Autodesk Inventor part; units mm, degrees
ref_plane "Work Plane3" through (0, 0, 250) normal (0, 0, 1) x (1, 0, 0)
ref_plane "Start Plane" through (0, 0, 0) normal (0, 0, 1) x (1, 0, 0)
ref_plane "End Plane" through (0, 0, 450) normal (0, 0, 1) x (1, 0, 0)
sketch "Sketch" plane through (0, 0, 0) normal (0, 0, 1) x (1, 0, 0)
  line L0 (-13, 15) -> (13, 15)
  line L1 (15, 13) -> (15, -13)
  line L2 (-15, 15) -> (15, -15) construction
  line L3 (15, 15) -> (-15, -15) construction
  line L4 (-5.2, 15) -> (-5.2, 14.2)
  line L5 (-5.2, 14.2) -> (-4.1, 14.2)
  line L6 (-4.1, 14.2) -> (-4.1, 12.2)
  line L7 (-4.1, 12.2) -> (-8.25, 12.2)
  line L8 (-8.25, 12.2) -> (-8.25, 10.2)
  line L9 (-8.25, 10.2) -> (-3.85, 5.8)
  line L10 (-3.85, 5.8) -> (3.85, 5.8)
  line L11 (8.25, 12.2) -> (4.1, 12.2)
  line L12 (4.1, 12.2) -> (4.1, 14.2)
  line L13 (4.1, 14.2) -> (5.2, 14.2)
  line L14 (5.2, 14.2) -> (5.2, 15)
  line L15 (8.25, 12.2) -> (8.25, 10.2)
  line L16 (8.25, 10.2) -> (3.85, 5.8)
  line L17 (-2.5, 0) -> (0, 0)
  line L18 (-5.2, -15) -> (-5.2, -14.2)
  line L19 (-5.2, -14.2) -> (-4.1, -14.2)
  line L20 (-4.1, -14.2) -> (-4.1, -12.2)
  line L21 (-4.1, -12.2) -> (-8.25, -12.2)
  line L22 (-8.25, -12.2) -> (-8.25, -10.2)
  line L23 (-8.25, -10.2) -> (-3.85, -5.8)
  line L24 (-3.85, -5.8) -> (3.85, -5.8)
  line L25 (8.25, -12.2) -> (4.1, -12.2)
  line L26 (4.1, -12.2) -> (4.1, -14.2)
  line L27 (4.1, -14.2) -> (5.2, -14.2)
  line L28 (5.2, -14.2) -> (5.2, -15)
  line L29 (8.25, -12.2) -> (8.25, -10.2)
  line L30 (8.25, -10.2) -> (3.85, -5.8)
  line L31 (15, 5.2) -> (14.2, 5.2)
  line L32 (14.2, 5.2) -> (14.2, 4.1)
  line L33 (14.2, 4.1) -> (12.2, 4.1)
  line L34 (12.2, 4.1) -> (12.2, 8.25)
  line L35 (15, -5.2) -> (14.2, -5.2)
  line L36 (14.2, -5.2) -> (14.2, -4.1)
  line L37 (14.2, -4.1) -> (12.2, -4.1)
  line L38 (12.2, -4.1) -> (12.2, -8.25)
  line L39 (12.2, -8.25) -> (10.2, -8.25)
  line L40 (10.2, -8.25) -> (5.8, -3.85)
  line L41 (5.8, -3.85) -> (5.8, 3.85)
  line L42 (5.8, 3.85) -> (10.2, 8.25)
  line L43 (10.2, 8.25) -> (12.2, 8.25)
  line L44 (-15, 5.2) -> (-14.2, 5.2)
  line L45 (-14.2, 5.2) -> (-14.2, 4.1)
  line L46 (-14.2, 4.1) -> (-12.2, 4.1)
  line L47 (-12.2, 4.1) -> (-12.2, 8.25)
  line L48 (-15, -5.2) -> (-14.2, -5.2)
  line L49 (-14.2, -5.2) -> (-14.2, -4.1)
  line L50 (-14.2, -4.1) -> (-12.2, -4.1)
  line L51 (-12.2, -4.1) -> (-12.2, -8.25)
  line L52 (-12.2, -8.25) -> (-10.2, -8.25)
  line L53 (-10.2, -8.25) -> (-5.8, -3.85)
  line L54 (-5.8, -3.85) -> (-5.8, 3.85)
  line L55 (-5.8, 3.85) -> (-10.2, 8.25)
  line L56 (-10.2, 8.25) -> (-12.2, 8.25)
  circle A0 centre (11.5, 11.5) radius 1.65
  circle A1 centre (11.5, -11.5) radius 1.65
  circle A2 centre (-11.5, 11.5) radius 1.65
  circle A3 centre (-11.5, -11.5) radius 1.65
  line L57 (-15, -13) -> (-15, -5.2)
  line L58 (-15, 5.2) -> (-15, 13)
  line L59 (13, -15) -> (5.2, -15)
  line L60 (-5.2, -15) -> (-13, -15)
  arc A4 (-13, 15) -> (-15, 13) centre (-13, 13) ccw
  arc A5 (15, 13) -> (13, 15) centre (13, 13) ccw
  arc A6 (13, -15) -> (15, -13) centre (13, -13) ccw
  arc A7 (-15, -13) -> (-13, -15) centre (-13, -13) ccw
  circle A8 centre (0, 0) radius 2.5
  point P0 (0, 0)
  point P1 (0, 5.8)
  point P2 (0, -2.5)
  point P3 (0, 2.5)
  dimension "d2" = 8.2
  dimension "d3" = 4.1
  dimension "d4" = 10.4
  dimension "d5" = 5.2
  dimension "d8" = 9.2
  dimension "d11" = 16.5
  dimension "d12" = 8.25
  dimension "d14" = 0.8
  dimension "d15" = 2
  dimension "d16" = 2
  dimension "d34" = 0.8
  dimension "d35" = 10.4
  dimension "d36" = 5.2
  dimension "d37" = 8.2
  dimension "d38" = 4.1
  dimension "d39" = 2
  dimension "d40" = 16.5
  dimension "d41" = 8.25
  dimension "d42" = 2
  dimension "d43" = 9.2
  dimension "d44" = 23
  dimension "d45" = 11.5
  dimension "d46" = 23
  dimension "d48" = 3.3
  dimension "d55" = 2
  dimension "d62" = 5
  dimension "d65" = 11.5
  dimension "d66" = 6.4
  dimension "d67" = 3.25
  dimension "d68" = 4.15
  dimension "d69" = 0.8
  dimension "d70" = 2
  dimension "d71" = 2.7577
  dimension "d72" = 5.8
  dimension "d73" = 2.7577
  dimension "d74" = 4.15
  dimension "d75" = 2
  dimension "d76" = 3.25
  dimension "d77" = 2
  dimension "d78" = 1.1
  dimension "d79" = 0.8
  dimension "d80" = 135
  dimension "d81" = 2
  dimension "d82" = 1.1
  dimension "d83" = 7.4
  dimension "d84" = 7.4
  dimension "d85" = 6.4
  dimension "d86" = 6.3
ref_plane "Work Plane3" through (0, 0, 250) normal (0, 0, 1) x (1, 0, 0)
ref_plane "Start Plane" through (0, 0, 0) normal (0, 0, 1) x (1, 0, 0)
ref_plane "End Plane" through (0, 0, 450) normal (0, 0, 1) x (1, 0, 0)
ref_plane "Start Plane1" through (0, 0, 0) normal (0, 0, 1) x (1, 0, 0)
ref_plane "End Plane1" through (0, 0, 450) normal (0, 0, 1) x (1, 0, 0)
ref_plane "Start Plane2" through (0, 0, 15) normal (0, 0, 1) x (1, 0, 0)
ref_plane "End Plane2" through (0, 0, 435) normal (0, 0, 1) x (1, 0, 0)
extrude "Body" add sketch "Sketch" along normal up to surface (420 mm away) from surface at 15 contours L0 L4 L5 L6 L7 L8 L9 L10 L16 L15 L11 L12 L13 L14 A5 L1 L31 L32 L33 L34 L43 L42 L41 L40 L39 L38 L37 L36 L35 A6 L59 L28 L27 L26 L25 L29 L30 L24 L23 L22 L21 L20 L19 L18 L60 A7 L57 L48 L49 L50 L51 L52 L53 L54 L55 L56 L47 L46 L45 L44 L58 A4
sketch "Sketch7" plane through (0, 0, 0) normal (0, 0, 1) x (1, 0, 0)
  line L0 (0, 0) -> (10, 0)
ref_plane "Work Plane10" through (0, 0, 0) normal (0, -1, 0) x (1, 0, 0)
sketch "Sketch8" plane through (0, 0, 0) normal (0, -1, 0) x (1, 0, 0)
  line L0 (-2, 15) -> (12, 15)
  line L1 (-2, 435) -> (12, 435)
  dimension "d100" = 420
ref_plane "Work Plane11" through (-225, 5.2, 435) normal (0, 0, 1) x (1, 0, 0)
split "Split1" plane through (-225, 5.2, 435) removes the side toward (0, 0, 1)
ref_plane "Work Plane12" through (225, -13, 15) normal (0, 0, -1) x (-1, 0, 0)
split "Split2" plane through (225, -13, 15) removes the side toward (0, 0, -1)
equation "\"d38\" = 0.5 * d37"
equation "\"d41\" = 0.5 * d40"
equation "\"d45\" = 0.5 * d44"
equation "\"G_OFFSET_START\" = 0"
equation "\"G_OFFSET_END\" = 0"
equation "\"G_L\" = 500"
equation "\"G_OFFSET_START1\" = 0"
equation "\"G_OFFSET_END1\" = 0"
equation "\"G_OFFSET_START2\" = -15"
equation "\"G_OFFSET_END2\" = -15"
equation "\"d95\" = -G_OFFSET_START2"
equation "\"d96\" = Length + G_OFFSET_END2"
properties part number "420 mm" material "Aluminum 6061"
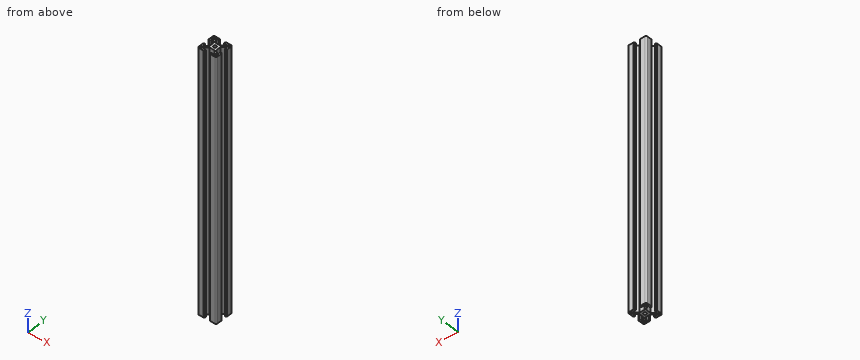
The model under review builds one solid part; all positions refer to its coordinate system, in mm. Coordinates: 2 decimals unless noted, no trailing zeros. Answer in a Markdown table with one row per item. Add a question column.
Item 1: To check wall thickness, follow probe 1 along Y at (x, z) = (11.5, 178); probe 2 along X at (y, z) = (0, 271); probe 3 along X at (y, z) = (11.75, 97). State the ranges of each line that lie inside material, in increasing order.
Item 2: We need section A-A on z = 292. Give the number of separate pieces and of enclosed holes in the cut face, plus the area to 3 significant figures.
Item 3: Clearance check with flat-ended pins moving along their axes: pin 1 (0.6 mm diameter, centred on x = 14.5, z = 144, fed in from +Y); pin 2 (0.6 mm diameter, centred on y = 4.5, z = 134, fed in from -X); pin 3 (3 mm diameter, centred on x = 3.5, z = 360.5, fed in from +Y). State where each tip first meets the part, or that it passes through.
Final values:
| question | item | result |
|---|---|---|
| 1 | probe 1 | y = -15 to -13.15, -9.85 to -8.25, 8.25 to 9.85, 13.15 to 15 |
| 1 | probe 2 | x = -5.8 to -2.5, 2.5 to 5.8 |
| 1 | probe 3 | x = -15 to -13.13, -9.87 to -8.25, 8.25 to 9.87, 13.13 to 15 |
| 2 | separate pieces | 1 |
| 2 | enclosed holes | 5 |
| 2 | area | 399 mm2 |
| 3 | pin 1 | stops at y = 14.6 |
| 3 | pin 2 | stops at x = -14.2 |
| 3 | pin 3 | stops at y = 14.2 |
